```python
from build123d import *

# Parameters (mm, degrees)
F0_R     = 1.15
F1_DEPTH = 2
F2_DEPTH = 105
F4_R     = 2.75
F4_R_2   = 1.75
F5_DEPTH = 2
F6_DEPTH = 2
F8_R     = 1.15
F9_DEPTH = 18


with BuildPart() as f1:
    # F0 (on Top) → F1 (new body)
    with BuildSketch(Plane.XY):
        with BuildLine():
            ThreePointArc((0, 2.8), (0.8201010127, 0.8201010127), (2.8, 0))
            Line((2.8, 0), (84.2, 0))
            ThreePointArc((84.2, 0), (86.1798989873, 0.8201010127), (87, 2.8))
            Line((87, 2.8), (87, 53.2))
            ThreePointArc((87, 53.2), (86.1798989873, 55.1798989873), (84.2, 56))
            Line((84.2, 56), (2.8, 56))
            ThreePointArc((2.8, 56), (0.8201010127, 55.1798989873), (0, 53.2))
            Line((0, 53.2), (0, 2.8))
        make_face()
        with Locations((3.5, 3.5)):
            Circle(F0_R, mode=Mode.SUBTRACT)
        with Locations((61.5, 3.5)):
            Circle(F0_R, mode=Mode.SUBTRACT)
        with Locations((3.5, 52.5)):
            Circle(F0_R, mode=Mode.SUBTRACT)
        with Locations((61.5, 52.5)):
            Circle(F0_R, mode=Mode.SUBTRACT)
        with Locations((3.5, 3.5)):
            Circle(F0_R)
        with Locations((61.5, 52.5)):
            Circle(F0_R)
        with Locations((61.5, 3.5)):
            Circle(F0_R)
        with Locations((3.5, 52.5)):
            Circle(F0_R)
    extrude(amount=F1_DEPTH)

    # F0 (on Top) → F2 (join)
    with BuildSketch(Plane.XY):
        with Locations((61.5, 3.5)):
            Circle(F0_R)
        with Locations((61.5, 52.5)):
            Circle(F0_R)
        with Locations((3.5, 52.5)):
            Circle(F0_R)
        with Locations((3.5, 3.5)):
            Circle(F0_R)
    extrude(amount=F2_DEPTH)


with BuildPart() as f5:
    # F4 (on offset) → F5 (new body)
    with BuildSketch(Plane.XY.offset(25)):
        with BuildLine():
            Line((84.2, 56), (2.8, 56))
            ThreePointArc((2.8, 56), (0.8201010127, 55.1798989873), (0, 53.2))
            Line((0, 53.2), (0, 2.8))
            ThreePointArc((0, 2.8), (0.8201010127, 0.8201010127), (2.8, 0))
            Line((2.8, 0), (84.2, 0))
            ThreePointArc((84.2, 0), (86.1798989873, 0.8201010127), (87, 2.8))
            Line((87, 2.8), (87, 53.2))
            ThreePointArc((87, 53.2), (86.1798989873, 55.1798989873), (84.2, 56))
        make_face()
        with Locations((3.5, 3.5)):
            Circle(F4_R, mode=Mode.SUBTRACT)
        with Locations((61.5, 3.5)):
            Circle(F4_R, mode=Mode.SUBTRACT)
        with Locations((3.5, 52.5)):
            Circle(F4_R, mode=Mode.SUBTRACT)
        with Locations((61.5, 52.5)):
            Circle(F4_R, mode=Mode.SUBTRACT)
        with Locations((3.5, 3.5)):
            Circle(F4_R)
        with Locations((3.5, 3.5)):
            Circle(F4_R_2, mode=Mode.SUBTRACT)
        with Locations((61.5, 3.5)):
            Circle(F4_R)
        with Locations((61.5, 3.5)):
            Circle(F4_R_2, mode=Mode.SUBTRACT)
        with Locations((61.5, 52.5)):
            Circle(F4_R)
        with Locations((61.5, 52.5)):
            Circle(F4_R_2, mode=Mode.SUBTRACT)
        with Locations((3.5, 52.5)):
            Circle(F4_R)
        with Locations((3.5, 52.5)):
            Circle(F4_R_2, mode=Mode.SUBTRACT)
        with Locations((3.5, 3.5)):
            Circle(F4_R_2)
        with Locations((61.5, 3.5)):
            Circle(F4_R_2)
        with Locations((61.5, 52.5)):
            Circle(F4_R_2)
        with Locations((3.5, 52.5)):
            Circle(F4_R_2)
    extrude(amount=F5_DEPTH)

    # F4 (on offset) → F6 (join, through all)
    with BuildSketch(Plane.XY.offset(25)):
        with Locations((3.5, 3.5)):
            Circle(F4_R)
        with Locations((3.5, 3.5)):
            Circle(F4_R_2, mode=Mode.SUBTRACT)
        with Locations((3.5, 52.5)):
            Circle(F4_R)
        with Locations((3.5, 52.5)):
            Circle(F4_R_2, mode=Mode.SUBTRACT)
        with Locations((61.5, 52.5)):
            Circle(F4_R)
        with Locations((61.5, 52.5)):
            Circle(F4_R_2, mode=Mode.SUBTRACT)
        with Locations((61.5, 3.5)):
            Circle(F4_R)
        with Locations((61.5, 3.5)):
            Circle(F4_R_2, mode=Mode.SUBTRACT)
    extrude(amount=F6_DEPTH)

    # F8 (on face) → F9 (join)
    with BuildSketch(Plane.XY.offset(27)):
        with Locations((3.5, 52.5)):
            Circle(F8_R)
        with Locations((61.5, 52.5)):
            Circle(F8_R)
        with Locations((61.5, 3.5)):
            Circle(F8_R)
        with Locations((3.5, 3.5)):
            Circle(F8_R)
    extrude(amount=F9_DEPTH)


solid = f5.part
```
For this review, take the finished solid that the model builds, in its own axes (mm). A direction names the side the tool comes from. Round coordinates to 2 decimals unless told otherwise and drop trailing zeros. Write each loop counter-clockwise with the first axis right and the second up, starting at its lowest first coordinate (ties: lowest second). Pieces come first, ordered by that corner, then holes. Notation, with made-up numbers: (-15, -29.75) -> (32, -29.75) arc R16 ccw to (32, -24.75) -> close; hole circle Ø3 at (-3, 59.25). An arc over 180 degrees is marked (long way). Use one line per item in the form item = value.
1) Take a section at A-A, the plane z = 33.5. Write out the cut boundary in (x, y).
Found:
outline = circle Ø2.3 at (3.5, 3.5); circle Ø2.3 at (3.5, 52.5); circle Ø2.3 at (61.5, 3.5); circle Ø2.3 at (61.5, 52.5)
2) Take a section at D-D, the plane x = 77.5. Write out the cut boundary in (y, z).
Found:
outline = (0, 25) -> (56, 25) -> (56, 27) -> (0, 27) -> close
3) Tool access review of faces 4 (the flat face through (61, 4, 45)), 5 (the cylindrical face through (3.251, 51.377, 35.874)): name each direction out of +Z, -Z, +X, -X, +Y, -Y from which nothing blocks a thin tool from reaching the whole face with its end or side.
Found:
face_4 = +Z, +X, -X, +Y, -Y
face_5 = +Z
4) Take a section at C-C, the plane y = 44. Write out the cut boundary in (x, z), and give its area (3 significant figures).
Found:
outline = (0, 25) -> (87, 25) -> (87, 27) -> (0, 27) -> close
area = 174 mm2
5) Mouldability with a two-part tool opening along X and no side actions: class faces 1 (the cylindrical face through (86.2, 55.16, 25.99)), 2 (the cylindrical face through (62.597, 52.845, 35.874)), 3 (the flat face through (43, 28, 25)) as +X half, -X half, draft (parallel to the pull), parting line (faces both ways), or undercut.
Found:
face_1 = +X half
face_2 = undercut
face_3 = draft
6) Clearance check with a flat-ended pin moving along its axis: pin 1 (10 mm diameter, centred on x = 16, y = 46.5, fed in from +Z). State where the tip first meets the part, or that it passes through.
Found:
pin_1 = 27
7) Take a section at B-B, the plane x = 61.5. Write out the cut boundary in (y, z), and give its area (3 significant figures).
Found:
outline = (0, 25) -> (56, 25) -> (56, 27) -> (53.65, 27) -> (53.65, 45) -> (51.35, 45) -> (51.35, 27) -> (4.65, 27) -> (4.65, 45) -> (2.35, 45) -> (2.35, 27) -> (0, 27) -> close
area = 195 mm2
8) To check wall thickness, follow L1, parallel to Z at x = 13.5, y = 28.5; L2, parallel to Y at x = 4, z = 27.25. State the ranges of each line that lie inside material, in increasing order. Write a range as from..to.
Found:
L1 = 25..27
L2 = 2.46..4.54, 51.46..53.54
